from build123d import *

# Parameters (mm, degrees)
SKETCH3_W           = 44.45
SKETCH3_H           = 25.4
BOSS_EXTRUDE2_DEPTH = 9.525
SKETCH4_W           = 34.925
SKETCH4_H           = 15.875
CUT_EXTRUDE1_DEPTH  = 10.525
SKETCH5_R           = 1.143
CUT_EXTRUDE2_DEPTH  = 9.525
SKETCH6_W           = 34.925
SKETCH6_H           = 9.525
CUT_EXTRUDE3_DEPTH  = 3.175
SKETCH7_W           = 19.05
SKETCH7_H           = 3.81
CUT_EXTRUDE4_DEPTH  = 26.4
FILLET1_R           = 3.175
SKETCH8_R           = 1.143
SKETCH8_R_2         = 1.41354867
CUT_EXTRUDE5_DEPTH  = 9.525
SKETCH9_W           = 9.525
SKETCH9_H           = 25.4
SKETCH9_R           = 1.143
BOSS_EXTRUDE3_DEPTH = 2.54
SKETCH10_W          = 9.525
SKETCH10_H          = 19.05
SKETCH10_R          = 1.143
CUT_EXTRUDE6_DEPTH  = 5.715


with BuildPart() as part:
    # Sketch3 → Boss-Extrude2 (new body)
    with BuildSketch(Plane.XY):
        with Locations((-22.225, 12.7)):
            Rectangle(SKETCH3_W, SKETCH3_H)
    extrude(amount=BOSS_EXTRUDE2_DEPTH)

    # Sketch4 → Cut-Extrude1 (cut, through all)
    with BuildSketch(Plane.XY.offset(9.525)):
        with Locations((-26.9875, 7.9375)):
            Rectangle(SKETCH4_W, SKETCH4_H)
    extrude(amount=-CUT_EXTRUDE1_DEPTH, mode=Mode.SUBTRACT)

    # Sketch5 → Cut-Extrude2 (cut)
    with BuildSketch(Plane(origin=(0, 0, 0), x_dir=(0, 0, -1), z_dir=(1, 0, 0))):
        with Locations((-4.7625, 3.175)):
            Circle(SKETCH5_R)
        with Locations((-4.7625, 15.875)):
            Circle(SKETCH5_R)
    extrude(amount=-CUT_EXTRUDE2_DEPTH, mode=Mode.SUBTRACT)

    # Sketch6 → Cut-Extrude3 (cut)
    with BuildSketch(Plane.XZ.offset(-15.875)):
        with Locations((-26.9875, 4.7625)):
            Rectangle(SKETCH6_W, SKETCH6_H)
    extrude(amount=-CUT_EXTRUDE3_DEPTH, mode=Mode.SUBTRACT)

    # Sketch7 → Cut-Extrude4 (cut, through all)
    with BuildSketch(Plane(origin=(0, 25.4, 0), x_dir=(1, 0, 0), z_dir=(0, 1, 0))):
        with Locations((-22.225, -1.905)):
            Rectangle(SKETCH7_W, SKETCH7_H)
    extrude(amount=-CUT_EXTRUDE4_DEPTH, mode=Mode.SUBTRACT)

    # Fillet1
    fillet1_edges = [part.edges().sort_by_distance(p)[0] for p in [
        (-12.7, 22.225, 3.81),
        (-31.75, 22.225, 3.81),
    ]]
    fillet(fillet1_edges, radius=FILLET1_R)

    # Sketch8 → Cut-Extrude5 (cut)
    with BuildSketch(Plane(origin=(0, 25.4, 0), x_dir=(1, 0, 0), z_dir=(0, 1, 0))):
        with Locations((-39.6875, -4.7625)):
            Circle(SKETCH8_R)
        with Locations((-4.7625, -4.7625)):
            Circle(SKETCH8_R_2)
    extrude(amount=-CUT_EXTRUDE5_DEPTH, mode=Mode.SUBTRACT)

    # Sketch9 → Boss-Extrude3 (add)
    with BuildSketch(Plane(origin=(0, 0, 0), x_dir=(0, 0, -1), z_dir=(1, 0, 0))):
        with Locations((-4.7625, 12.7)):
            Rectangle(SKETCH9_W, SKETCH9_H)
        with Locations((-4.7625, 15.875)):
            Circle(SKETCH9_R, mode=Mode.SUBTRACT)
        with Locations((-4.7625, 3.175)):
            Circle(SKETCH9_R, mode=Mode.SUBTRACT)
    extrude(amount=BOSS_EXTRUDE3_DEPTH)

    # Sketch10 → Cut-Extrude6 (cut)
    with BuildSketch(Plane.ZY.offset(9.525)):
        with Locations((4.7625, 9.525)):
            Rectangle(SKETCH10_W, SKETCH10_H)
        with Locations((4.7625, 15.875)):
            Circle(SKETCH10_R, mode=Mode.SUBTRACT)
        with Locations((4.7625, 3.175)):
            Circle(SKETCH10_R, mode=Mode.SUBTRACT)
    extrude(amount=-CUT_EXTRUDE6_DEPTH, mode=Mode.SUBTRACT)


solid = part.part
Geometry check sheet. Reference: the model listing, model coordinates, mm. A direction names the side the tool comes from. Round coordinates to 2 decimals unless told otherwise and drop trailing zeros. Order: outer loops, then holes, each group sorted by start corner. A loop starts at its lowest first (then second) coordinate and runs counter-clockwise, first axis right, second up. Notation, with made-up numbers: (-18, -3.5) - (41, -3.5) arc R17 ccw to (41, 15.5) - close; hole circle Ø2 at (87, 88). An arc over 180 degrees is marked (long way). One line per question, with ' | ' between items. Start each with the question number.
(1) Sectioned sample at D-D on y = 8.75. Record the cut outline in (x, z) (3 decimals), and give its area (3 significant figures).
(2) Sectioned sample at C-C on z = 1.25. Record the cut outline in (x, y), and give its area (3 significant figures).
(3) Depth check by flat-ended pin: pin 1 Ø1.9 at (x, y) = (-20, 23.5) entering from -Z; pin 2 Ø2.5 at (y, z) = (15.88, 4.76) entering from +X; pin 3 Ø3.5 at (y, z) = (15.88, 4.76) entering from -X; pin 4 Ø3.5 at (x, z) = (-39.69, 4.76) entering from -Y. Enter the tip coordinate at first touch or a pass-through.
(4) Access from +Z, -Z, +X, -X, +Y, -Y to the whole of each face (thin tool, end or side, straight path). Record for faces 4 (the flat face through (-22, 22, 3.81)), 5 (the cylindrical face through (-3.457, 21.94, 5.304)), 6 (the flat face through (-3.81, 10, 5)).
(5) Sectioned sample at A-A on z = 5.25. Record the cut outline in (x, y), and give its area (3 significant figures).
(6) Thickness scan on L1, parallel to Y at x = -7, z = 6.75; L2, parallel to X at y = 4.25, z = 4; L3, parallel to Z at x = -18.5, y = 20 (3 decimals). Record the ranges inside material, lowest first. Write a range as [from, to].
(7) Sectioned sample at B-B on z = 8.75. Record the cut outline in (x, y), and give its area (3 significant figures).
(8) Release check for a two-part mould opening along Z. For faces 1 (the flat face through (-24, 19.05, 6)), 2 (the flat face through (-38, 22, 0)), 3 (the cylindrical face through (-40.53, 22.27, 3.99)) record: released by +Z, released by -Z, zero draft, split by the parting line, or undercut.
Conclusion:
1) outline: (-3.81, 0) - (2.54, 0) - (2.54, 9.525) - (-3.81, 9.525) - close | area: 60.5 mm2
2) outline: (-44.45, 19.05) - (-31.69, 19.05) - (-31.69, 25.4) - (-44.45, 25.4) - close; (-12.76, 19.05) - (-3.81, 19.05) - (-3.81, 0) - (2.54, 0) - (2.54, 25.4) - (-12.76, 25.4) - close | area: 299 mm2
3) pin 1: stops at z = 3.81 | pin 2: stops at x = 2.54 | pin 3: stops at x = -3.81 | pin 4: stops at y = 19.05
4) face 4: -Z, +Y, -Y | face 5: +Y | face 6: +Z, -Z, -X, -Y
5) outline: (-44.45, 19.05) - (-40.72, 19.05) - (-40.72, 25.4) - (-44.45, 25.4) - close; (-38.65, 19.05) - (-6.09, 19.05) - (-6.09, 25.4) - (-38.65, 25.4) - close; (-3.81, 0) - (2.54, 0) - (2.54, 2.14) - (-3.81, 2.14) - close; (-3.81, 4.21) - (2.54, 4.21) - (2.54, 14.84) - (-3.81, 14.84) - close; (-3.44, 16.91) - (2.54, 16.91) - (2.54, 25.4) - (-3.44, 25.4) - close | area: 362 mm2
6) L1: y = [19.05, 25.4] | L2: x = [-3.81, 2.54] | L3: z = [3.81, 9.525]
7) outline: (-44.45, 19.05) - (-3.81, 19.05) - (-3.81, 0) - (2.54, 0) - (2.54, 25.4) - (-44.45, 25.4) - close | area: 419 mm2
8) face 1: zero draft | face 2: released by -Z | face 3: undercut
